The model under review builds one solid part; all positions refer to its coordinate system, in mm. Face numbers are marked on the shaded views. Round coordinates to 2 decimals unless told otherwise and drop trailing zeros. Loops run counter-clockwise (first coordinate to the right, second up) from the corner with the lowest first, then second, coordinate; pieces in that order, holes last. Notation, with made-up numbers: M 70.25,44 L 114.25,44 A16 cw 114.25,53 Z; hole C -20.75,47 d2. An arc over 180 degrees is marked long. Return JSON: item names as keys, results as strings. Group by question number.
Q1. Consider section C-C (y = 49). State the section outline as (x, z) points (3 decimals), and give its area (3 significant figures).
Q2. Consider section B-B (x = 105). State the section outline as (y, z) points (1 decimal), and give its area (3 significant figures).
Q3. Draft analysis for pull direction X (two halves, no side actions). For the marked faces 1, 2 and 3, state which applies: pulls with the +X half, pulls with the -X half, needs draft (parallel to the pull), parting line crosses it, or undercut.
Q4. Consider section D-D (z = 0.5). State the section outline as (x, y) points, and give its area (3 significant figures).
Q5. To check wall thickness, follow line 1 along Y through (x, z) = (105, 1.25); line 2 along X through (y, z) = (51, 1.5); line 3 along Y through (x, z) = (104.5, 1.5). State the ranges of each line that lie inside material, in increasing order.
Q6. Clearance check with flat-ended pins moving along their axes: pin 1 Ø4 at (x, y) = (95.98, 52.01) entering from +Z (3 decimals); pin 2 Ø8 at (x, y) = (83.5, 44) entering from -Z; pin 3 Ø3 at (y, z) = (45, -1.5) entering from +X; pin 4 Ø3 at (x, z) = (105, -1) entering from -Y. State where each tip first meets the part, or that it passes through.
Q7. Consider section A-A (x = 96.5). State the section outline as (y, z) points (1 decimal), and give its area (3 significant figures).
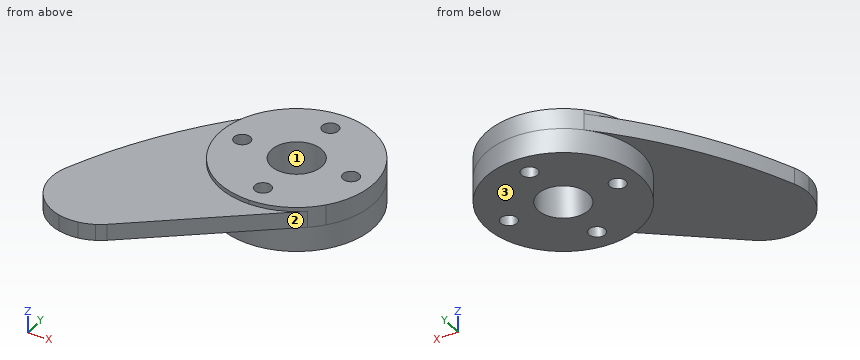
from build123d import *
from build123d.topology import SkipClean

# Parameters (mm, degrees)
SKETCH1_R           = 12
BOSS_EXTRUDE1_DEPTH = 3.175
BOSS_EXTRUDE2_START = 3.81
SKETCH2_R           = 12
BOSS_EXTRUDE2_DEPTH = 3.81
SKETCH3_R           = 3.937
CUT_EXTRUDE1_DEPTH  = 134.099089527
SKETCH4_R           = 1.27
CUT_EXTRUDE2_DEPTH  = 134.099089527
CUT_EXTRUDE3_DEPTH  = 133.970273023
CUT_EXTRUDE4_START  = -0.635
CUT_EXTRUDE4_DEPTH  = 0.635
BOSS_EXTRUDE3_START = -2.54
BOSS_EXTRUDE3_DEPTH = 2.54


with BuildPart() as part:
    # Sketch1 → Boss-Extrude1 (new body)
    with BuildSketch(Plane.XY):
        with BuildLine():
            ThreePointArc((79.156979953, 34.616777747), (78.764409425, 33.207913627), (78.648230314, 31.75))
            Line((78.648230314, 31.75), (93.886132052, 31.75))
            ThreePointArc((93.886132052, 31.75), (93.886918896, 31.813218964), (93.887181183, 31.876442281))
            ThreePointArc((93.887181183, 31.876442281), (87.66085737, 39.367908538), (79.156979953, 34.616777747))
        make_face()
        with BuildLine():
            ThreePointArc((87.4395, 24.347161532), (88.598049964, 24.621688616), (89.699693339, 25.073335615))
            ThreePointArc((89.699693339, 25.073335615), (92.723044454, 27.828451492), (93.886132052, 31.75))
            Line((93.886132052, 31.75), (78.648230314, 31.75))
            ThreePointArc((78.648230314, 31.75), (79.141141445, 29.177561465), (80.476005529, 26.924))
            Line((80.476005529, 26.924), (87.4395, 26.924))
            Line((87.4395, 26.924), (87.4395, 24.347161532))
        make_face()
        with BuildLine():
            Line((87.4395, 26.924), (80.476005529, 26.924))
            ThreePointArc((80.476005529, 26.924), (82.246043304, 25.403819152), (84.393093646, 24.490496444))
            ThreePointArc((84.393093646, 24.490496444), (85.909052633, 24.264862685), (87.4395, 24.347161532))
            Line((87.4395, 24.347161532), (87.4395, 26.924))
        make_face()
        with BuildLine():
            ThreePointArc((89.699693339, 25.073335615), (94.483227873, 27.711788353), (99.06, 30.694537484))
            Line((99.06, 30.694537484), (99.06, 31.75))
            Line((99.06, 31.75), (93.886132052, 31.75))
            ThreePointArc((93.886132052, 31.75), (92.723044454, 27.828451492), (89.699693339, 25.073335615))
        make_face()
        with BuildLine():
            ThreePointArc((99.06, 30.694537484), (106.888760949, 37.054762789), (113.784062988, 44.416608597))
            ThreePointArc((113.784062988, 44.416608597), (96.436063978, 43.110085278), (96.014300162, 60.502100346))
            ThreePointArc((96.014300162, 60.502100346), (86.225733854, 48.445051897), (79.156979953, 34.616777747))
            ThreePointArc((79.156979953, 34.616777747), (87.66085737, 39.367908538), (93.887181183, 31.876442281))
            ThreePointArc((93.887181183, 31.876442281), (93.886918896, 31.813218964), (93.886132052, 31.75))
            Line((93.886132052, 31.75), (99.06, 31.75))
            Line((99.06, 31.75), (99.06, 30.694537484))
        make_face()
        with Locations((104.48925, 52.0065)):
            Circle(SKETCH1_R)
    extrude(amount=BOSS_EXTRUDE1_DEPTH)

    # Sketch2 → Boss-Extrude2 (add)
    with SkipClean():  # the faces are left unmerged after this step: merging them gives an invalid solid
        with BuildSketch(Plane(origin=(0, 0, 0), x_dir=(-1, 0, 0), z_dir=(0, 0, -1)).offset(BOSS_EXTRUDE2_START)):
            with Locations((-104.48925, 52.0065)):
                Circle(SKETCH2_R)
        extrude(amount=-BOSS_EXTRUDE2_DEPTH)

    # Sketch3 → Cut-Extrude1 (cut, through all)
    with SkipClean():  # the faces are left unmerged after this step: merging them gives an invalid solid
        with BuildSketch(Plane(origin=(0, 0, -3.81), x_dir=(-1, 0, 0), z_dir=(0, 0, -1))):
            with Locations((-104.48925, 52.0065)):
                Circle(SKETCH3_R)
        extrude(amount=-CUT_EXTRUDE1_DEPTH, mode=Mode.SUBTRACT)

    # Sketch4 → Cut-Extrude2 (cut, through all)
    with SkipClean():  # the faces are left unmerged after this step: merging them gives an invalid solid
        with BuildSketch(Plane(origin=(0, 0, -3.81), x_dir=(-1, 0, 0), z_dir=(0, 0, -1))):
            with Locations((-112.99825, 52.0065)):
                Circle(SKETCH4_R)
            with Locations((-95.98025, 52.0065)):
                Circle(SKETCH4_R)
            with Locations((-104.48925, 60.5155)):
                Circle(SKETCH4_R)
            with Locations((-104.48925, 43.4975)):
                Circle(SKETCH4_R)
        extrude(amount=-CUT_EXTRUDE2_DEPTH, mode=Mode.SUBTRACT)

    # Sketch5 → Cut-Extrude3 (cut, through all)
    with SkipClean():  # the faces are left unmerged after this step: merging them gives an invalid solid
        with BuildSketch(Plane(origin=(0, 0, 0), x_dir=(-1, 0, 0), z_dir=(0, 0, -1))):
            with BuildLine():
                ThreePointArc((-104.430493989, 40.006643845), (-109.606684651, 41.15238269), (-113.7840634, 44.4166091))
                ThreePointArc((-113.7840634, 44.4166091), (-102.758092767, 33.479680706), (-89.699693406, 25.073335649))
                ThreePointArc((-89.699693406, 25.073335649), (-92.462895691, 27.440507008), (-93.81346398, 30.819079549))
                ThreePointArc((-93.81346398, 30.819079549), (-97.397477458, 37.40567327), (-104.430493989, 40.006643845))
            make_face()
        extrude(amount=-CUT_EXTRUDE3_DEPTH, mode=Mode.SUBTRACT)
    add(part.part.scale(1), mode=Mode.REPLACE)  # the faces are merged on a copy

    # Sketch6 → Cut-Extrude4 (cut)
    with BuildSketch(Plane.XY.offset(3.175).offset(CUT_EXTRUDE4_START)):
        with BuildLine():
            ThreePointArc((96.014299675, 60.502099861), (86.225733771, 48.44505177), (79.156980092, 34.616778107))
            ThreePointArc((79.156980092, 34.616778107), (84.355854315, 24.500045491), (93.81346398, 30.819079549))
            ThreePointArc((93.81346398, 30.819079549), (97.397477458, 37.40567327), (104.430493989, 40.006643845))
            ThreePointArc((104.430493989, 40.006643845), (93.388711037, 47.448207038), (96.014299675, 60.502099861))
        make_face()
    extrude(amount=CUT_EXTRUDE4_DEPTH, mode=Mode.SUBTRACT)

    # Sketch7 → Boss-Extrude3 (add)
    with BuildSketch(Plane.XY.offset(2.54).offset(BOSS_EXTRUDE3_START)):
        with BuildLine():
            ThreePointArc((93.81346398, 30.819079549), (92.885787929, 28.100406696), (91.017515109, 25.918361416))
            Line((91.017515109, 25.918361416), (111.970090828, 42.623695489))
            ThreePointArc((111.970090828, 42.623695489), (108.424231015, 40.670013577), (104.430493989, 40.006643845))
            ThreePointArc((104.430493989, 40.006643845), (97.397477458, 37.40567327), (93.81346398, 30.819079549))
        make_face()
    extrude(amount=BOSS_EXTRUDE3_DEPTH)


solid = part.part
Values:
{
 "1": {"outline": "M 86.591,0 L 92.872,0 L 92.872,-3.81 L 101.947,-3.81 L 101.947,3.175 L 92.872,3.175 L 92.872,2.54 L 86.591,2.54 Z; M 107.031,-3.81 L 116.107,-3.81 L 116.107,3.175 L 107.031,3.175 Z", "area": "143 mm2"},
 "2": {"outline": "M 37.1,0 L 40,0 L 40,-3.8 L 42.3,-3.8 L 42.3,3.2 L 40,3.2 L 40,2.5 L 37.1,2.5 Z; M 44.7,-3.8 L 48.1,-3.8 L 48.1,3.2 L 44.7,3.2 Z; M 55.9,-3.8 L 59.4,-3.8 L 59.4,3.2 L 55.9,3.2 Z; M 61.7,-3.8 L 64,-3.8 L 64,3.2 L 61.7,3.2 Z", "area": "88.0 mm2"},
 "3": {"face 1": "undercut", "face 2": "pulls with the +X half", "face 3": "needs draft"},
 "4": {"outline": "M 79.16,34.62 A7.62 ccw 91.02,25.92 L 111.97,42.62 A12 ccw long 96.01,60.5 A74.31 ccw Z; hole C 95.98,52.01 d2.54; hole C 104.49,52.01 d7.87; hole C 104.49,43.5 d2.54; hole C 104.49,60.52 d2.54; hole C 113,52.01 d2.54", "area": "815 mm2"},
 "5": {"line 1": "y = 37.07 to 42.33, 44.66 to 48.1, 55.91 to 59.35, 61.68 to 64", "line 2": "x = 87.97 to 95.21, 96.75 to 100.68, 108.3 to 112.22, 113.77 to 116.45", "line 3": "y = 36.67 to 42.23, 44.77 to 48.07, 55.94 to 59.25, 61.79 to 64.01"},
 "6": {"pin 1": "stops at z = 3.175", "pin 2": "stops at z = 0", "pin 3": "stops at x = 115.15", "pin 4": "stops at y = 36.18"},
 "7": {"outline": "M 30.3,0 L 43.1,0 L 43.1,-3.8 L 50.8,-3.8 L 50.8,3.2 L 43.1,3.2 L 43.1,2.5 L 30.3,2.5 Z; M 53.2,-3.8 L 61,-3.8 L 61,3.2 L 53.2,3.2 Z", "area": "141 mm2"}
}
